Autodesk Inventor part; units mm, degrees
ref_plane "YZ Plane" through (0, 0, 0) normal (1, 0, 0) x (0, 1, 0)
ref_plane "XZ Plane" through (0, 0, 0) normal (0, 1, 0) x (-1, 0, 0)
ref_plane "XY Plane" through (0, 0, 0) normal (0, 0, 1) x (1, 0, 0)
sketch "Sketch1" plane through (0, 0, 0) normal (0, 0, 1) x (1, 0, 0)
  circle A0 centre (0, 0) radius 2.2225
  dimension "d0" = 4.445
extrude "Extrusion1" add sketch "Sketch1" along normal mid plane 7.366
sketch "Sketch2" plane through (0, 0, 3.683) normal (0, 0, 1) x (1, 0, 0)
  circle A0 centre (0, 0) radius 2.2225
  circle A1 centre (0, 0) radius 4.064
  dimension "d3" = 8.128
extrude "Extrusion2" add sketch "Sketch2" along normal blind 1.778 contours A0 | A1
sketch "Sketch3" plane through (0, 0, -3.683) normal (0, 0, -1) x (-1, 0, 0)
  circle A0 centre (0, 0) radius 3.429
  dimension "d6" = 6.858
extrude "Extrusion3" add sketch "Sketch3" along normal blind 1.778
properties part number "Rivet" material "Stainless Steel"
The listing builds one solid part. Answer for the finished solid, in the listing's coordinates (mm). A direction names the side the tool comes from. Coordinates: 2 decimals unless noted, no trailing zeros. Write each loop counter-clockwise with the first axis right and the second up, starting at its lowest first coordinate (ties: lowest second). Pieces come first, ordered by that corner, then holes. Notation, with made-up numbers: (10.5, 45.5) - (30.5, 45.5) arc R32 cw to (30.5, 84.5) - close; hole circle Ø8 at (11, 86.25). An arc over 180 degrees is marked (long way). Return JSON: item names as keys, results as strings. Group by question number.
Q1. Flat-ended cylindrical pins translate along their axes: pin 1 Ø1 at (x, z) = (-0.5, -4) entering from +Y; pin 2 Ø4 at (y, z) = (1, -4) entering from +X; pin 3 Ø1.5 at (x, z) = (2, 3.5) entering from +Y. Find the tip coordinate at first contact, or state that the pin passes through.
Q2. The part is cut by section D-D on z = -1. Write down the section's boundary in (x, y) (1 decimal), and give its area (3 significant figures).
Q3. Find the intervals of material crossed by line 1 along Z through (x, y) = (-3, 1); line 2 along Y through (x, z) = (-1.5, 4); line 3 along X through (y, z) = (0.5, 1.5), in increasing order. Write a range as [from, to].
Q4. Which of the six approach directions +Z, -Z, +X, -X, +Y, -Y give full straight-line access (tool end or side, diameter ignored) to faces 5 (the cylindrical face through (-0.48, -2.17, 0.05)), 6 (the cylindrical face through (0.74, 3.35, -4.56))?
Q5. For a pull along Z with two mould halves and no side action, classify faces 1 (the flat face through (0, 0, 5.461)), 2 (the flat face through (2, 2, -3.683)), 3 (the flat face through (0, 0, -5.461)), 4 (the cylindrical face through (-0.881, 3.967, 4.56)) as +Z half, -Z half, draft (parallel to the pull), parting line (faces both ways), or undercut.
Q6. The part is cut by section B-B on x = 0. Write down the section's boundary in (y, z).
Q7. The part is cut by section A-A on y = 2.5. Write down the section's boundary in (x, z).
Evaluation:
{
 "1": {"pin 1": "stops at y = 3.43", "pin 2": "stops at x = 3.43", "pin 3": "stops at y = 3.86"},
 "2": {"outline": "circle Ø4.4 at (0, 0)", "area": "15.5 mm2"},
 "3": {"line 1": "z = [-5.46, -3.68], [3.68, 5.46]", "line 2": "y = [-3.78, 3.78]", "line 3": "x = [-2.17, 2.17]"},
 "4": {"face 5": "none", "face 6": "-Z"},
 "5": {"face 1": "+Z half", "face 2": "undercut", "face 3": "-Z half", "face 4": "draft"},
 "6": {"outline": "(-4.06, 3.68) - (-2.22, 3.68) - (-2.22, -3.68) - (-3.43, -3.68) - (-3.43, -5.46) - (3.43, -5.46) - (3.43, -3.68) - (2.22, -3.68) - (2.22, 3.68) - (4.06, 3.68) - (4.06, 5.46) - (-4.06, 5.46) - close"},
 "7": {"outline": "(-3.2, 3.68) - (3.2, 3.68) - (3.2, 5.46) - (-3.2, 5.46) - close; (-2.35, -5.46) - (2.35, -5.46) - (2.35, -3.68) - (-2.35, -3.68) - close"}
}
